```python
from build123d import *

# Parameters (mm, degrees)
SKETCH1_W           = 46
SKETCH1_H           = 70
BOSS_EXTRUDE1_DEPTH = 25
SKETCH2_R           = 12.5
BOSS_EXTRUDE2_DEPTH = 20
CUT_EXTRUDE1_REACH  = 89.413
SKETCH3_R           = 2.5


with BuildPart() as part:
    # Sketch1 → Boss-Extrude1 (new body)
    with BuildSketch(Plane(origin=(0, 0, 0), x_dir=(1, 0, 0), z_dir=(0, 1, 0))):
        with Locations((23, 35)):
            Rectangle(SKETCH1_W, SKETCH1_H)
    extrude(amount=BOSS_EXTRUDE1_DEPTH)

    # Sketch2 → Boss-Extrude2 (add)
    with BuildSketch(Plane.XY):
        with Locations(Location((23, 21.5, 0), (0, 0, 163.739795292))):
            Circle(SKETCH2_R)
    extrude(amount=BOSS_EXTRUDE2_DEPTH)

    # Sketch3 → Cut-Extrude1 (cut, up to next)
    with BuildSketch(Plane(origin=(0, 25, 0), x_dir=(1, 0, 0), z_dir=(0, 1, 0)), mode=Mode.PRIVATE) as cut_extrude1_sk1:
        with Locations(Location((3, 50, 0), (0, 0, 270))):
            Circle(SKETCH3_R)
    cut_extrude1_tool1 = extrude(cut_extrude1_sk1.sketch, amount=-CUT_EXTRUDE1_REACH, mode=Mode.PRIVATE) & part.part
    # Sketch3 → Cut-Extrude1 (cut, up to next)
    with BuildSketch(Plane(origin=(0, 25, 0), x_dir=(1, 0, 0), z_dir=(0, 1, 0)), mode=Mode.PRIVATE) as cut_extrude1_sk2:
        with Locations(Location((43, 50, 0), (0, 0, 270))):
            Circle(SKETCH3_R)
    cut_extrude1_tool2 = extrude(cut_extrude1_sk2.sketch, amount=-CUT_EXTRUDE1_REACH, mode=Mode.PRIVATE) & part.part
    add(cut_extrude1_tool1.solids().sort_by_distance((3, 25, -50))[0], mode=Mode.SUBTRACT)
    add(cut_extrude1_tool2.solids().sort_by_distance((43, 25, -50))[0], mode=Mode.SUBTRACT)


solid = part.part
```
Source: CAD feature listing. Evaluate the final solid. Frame: model axes, mm. A direction names the side the tool comes from. Round coordinates to 2 decimals unless told otherwise and drop trailing zeros. Loops run counter-clockwise (first coordinate to the right, second up) from the corner with the lowest first, then second, coordinate; pieces in that order, holes last. Notation, with made-up numbers: M -32,4.25 L 4,4.25 A14 cw 4,20.25 Z; hole C 70,-21 d10. An arc over 180 degrees is marked long. Put each result on its own line as item: value.
(1) Ray query, line 1 (X direction, y = 22.5, z = -50); line 2 (X direction, y = 9.5, z = -51); line 3 (Y direction, x = 26.5, z = -27). Return the intervals inside material, ascending. Write a range as [from, to].
Solutions:
line 1: [0, 0.5], [5.5, 40.5], [45.5, 46]
line 2: [0, 0.71], [5.29, 40.71], [45.29, 46]
line 3: [0, 25]
(2) Access query for faces 1 (the face through (23, 25, -35)), 2 (the face through (34.835, 17.476, 9.86)), 3 (the face through (0, 12, -35)). Directions: +Z, -Z, +X, -X, +Y, -Y. A direction counts if a zero-diameter tool reaches every point of the face in a straight line with its end or side. Return the directions, or none.
Solutions:
face 1: -Z, +X, -X, +Y
face 2: +Z
face 3: +Z, -Z, -X, +Y, -Y
(3) Section D-D, the plane x = 23. Return loops of the section in (y, z).
Solutions:
outline: M 0,-70 L 25,-70 L 25,0 L 34,0 L 34,20 L 9,20 L 9,0 L 0,0 Z
(4) Section A-A, the plane x = 3. Return loops of the section in (y, z), and give its area (4 significant figures).
Solutions:
outline: M 0,-70 L 25,-70 L 25,-52.5 L 0,-52.5 Z; M 0,-47.5 L 25,-47.5 L 25,0 L 0,0 Z
area: 1,625 mm²
(5) First-contact query: pin 1 (1.5 mm diameter, centred on x = 24.5, z = 1.5, fed in from +Y); pin 2 (14 mm diameter, centred on x = 23.5, z = -37, fed in from +Y); pin 3 (1.5 mm diameter, centred on x = 36.5, y = 23, fed in from +Z). Flat tips, straight axial feed; report the tip coordinate or a pass-through.
Solutions:
pin 1: y = 33.98
pin 2: y = 25
pin 3: z = 0
(6) Section B-B, the plane z = -50. Return loops of the section in (x, y), and give its area (3 significant figures).
Solutions:
outline: M 0,0 L 0.5,0 L 0.5,25 L 0,25 Z; M 5.5,0 L 40.5,0 L 40.5,25 L 5.5,25 Z; M 45.5,0 L 46,0 L 46,25 L 45.5,25 Z
area: 900 mm²
(7) Pull-direction query (X, two-part tool) for faces 4 (the face through (46, 12, -35)), 5 (the face through (24, 29, 0)), 6 (the face through (42.04, 12.68, -47.69)); classes: released by +X, released by -X, zero draft, split by the parting line, or undercut.
Solutions:
face 4: released by +X
face 5: zero draft
face 6: undercut
(8) Section C-C, the plane y = 21.5. Return loops of the section in (x, z), and give its area (3 significant figures).
Solutions:
outline: M 0,-70 L 46,-70 L 46,0 L 35.5,0 L 35.5,20 L 10.5,20 L 10.5,0 L 0,0 Z; hole C 3,-50 d5; hole C 43,-50 d5
area: 3,680 mm²
